from build123d import *

# Parameters (mm, degrees)
SKETCH4_R           = 36.068
BOSS_EXTRUDE1_DEPTH = 65.024
SKETCH5_R           = 21.463
BOSS_EXTRUDE2_DEPTH = 31.369


with BuildPart() as part:
    # Sketch1 → Revolve1 (revolve)
    with BuildSketch(Plane.XY, mode=Mode.PRIVATE) as revolve1_sk:
        Polygon((-70.612, -36.068), (-32.512, -36.068), (-32.512, -30.0863), (-70.612, -30.3149), align=None)
        Polygon((70.612, -30.3149), (32.512, -30.0863), (32.512, -36.068), (70.612, -36.068), align=None)
    revolve(revolve1_sk.sketch.rotate(Axis((-70.612, 0, 0), (1, 0, 0)), 270), axis=Axis((-70.612, 0, 0), (1, 0, 0)))



with BuildPart() as body_2:
    # Sketch2 → Revolve2 (revolve)
    with BuildSketch(Plane.XY):
        Polygon((16.8275, 59.944), (16.637, 31.369), (21.463, 31.369), (21.463, 59.944), align=None)
    revolve(axis=Axis((0, 0, 0), (0, 1, 0)))


with BuildPart() as part_1:
    add(part.part)

    add(body_2.part)  # Boss-Extrude1 merges body 2
    # Sketch4 → Boss-Extrude1 (add)
    with BuildSketch(Plane(origin=(-32.512, 0, 0), x_dir=(0, 0, -1), z_dir=(1, 0, 0))):
        with Locations(Location((0, 0, 0), (0, 0, 180))):
            Circle(SKETCH4_R)
    extrude(amount=BOSS_EXTRUDE1_DEPTH)

    # Sketch5 → Boss-Extrude2 (add)
    with BuildSketch(Plane.XZ.offset(-31.369)):
        Circle(SKETCH5_R)
    extrude(amount=BOSS_EXTRUDE2_DEPTH)

    # Sketch6 → Cut-Revolve1 (revolve, cut)
    with BuildSketch(Plane.XY, mode=Mode.PRIVATE) as cut_revolve1_sk:
        Polygon((-70.612, -30.3149), (-32.512, -30.0863), (-32.512, -24.6253), (32.512, -24.6253), (32.512, -30.0863), (70.612, -30.3149), (70.612, 0), (-70.612, 0), align=None)
    revolve(cut_revolve1_sk.sketch.rotate(Axis((70.612, 0, 0), (-1, 0, 0)), 270), axis=Axis((70.612, 0, 0), (-1, 0, 0)), mode=Mode.SUBTRACT)

    # Sketch7 → Cut-Revolve2 (revolve, cut)
    with BuildSketch(Plane.XY):
        Polygon((16.8275, 59.944), (16.637, 31.369), (12.1539, 31.369), (12.1539, 0), (0, 0), (0, 59.944), align=None)
    revolve(axis=Axis((0, 0, 0), (0, 1, 0)), mode=Mode.SUBTRACT)


solid = part_1.part
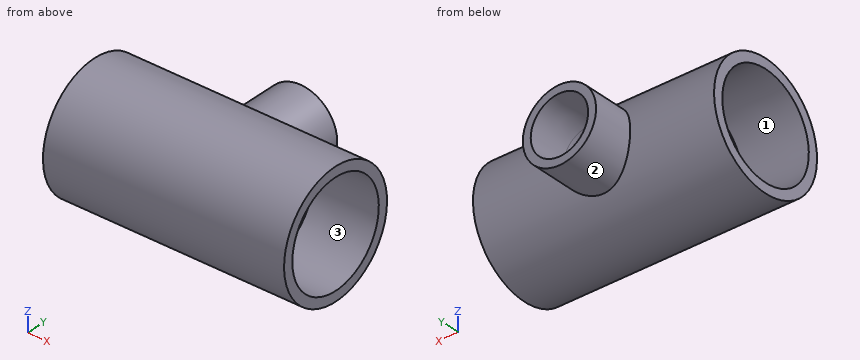
Can you work these out from the model? Positions are in its coordinate system, mm. Face numbers are marked on the shaded views. Coordinates: 2 decimals unless noted, no trailing zeros. Order: outer loops, then holes, each group sorted by start corner. A loop starts at its lowest first (then second) coordinate and runs counter-clockwise, first axis right, second up. Notation, with made-up numbers: (-24, 66) - (9, 66) arc R12 cw to (9, 72) - close; hole circle Ø10 at (-11, 80.5). An arc over 180 degrees is marked (long way). Answer as a JSON object with one key per item and string values. Group by question number.
Q1. I need wall thicknesses on line 1 (X direction, y = 26, z = 0); line 2 (Y direction, x = -11.5, z = 0); line 3 (Y direction, x = -36.5, z = 19). Which ranges of each line are inside material? Lowest first, please. Write a range as from..to.
Q2. Will these pins go through, and if not, where does the flat tip stop? P1, Ø5, axis at y = 9, z = -17.5, coming from the -X side (3 decimals); P2, Ø12, axis at x = 1.5, y = -17, coming from the +Z side; P3, Ø5, axis at x = 26.5, y = -13.5, coming from the -Z side; P4, Ø8, axis at x = -9, y = -6, coming from the -Z side.
Q3. We'd pull the mould along Z, two halves only. Please class the marked faces 1, 2 and 3: +Z half, -Z half, draft (parallel to the pull), parting line (faces both ways), or undercut.
Q4. Imagine slicing it at C-C (x = 35). Please give me the cut outline in (y, z).
Q5. Imagine slicing it at B-B (y = 46). Please give me the cut outline in (x, z), and give its area (3 significant figures).
Q6. Imagine slicing it at A-A (z = 0). Give the number of separate pieces and of enclosed holes in the cut face, and give its area (3 significant figures).
Determined:
{
 "1": {"line 1": "x = -32.51..-12.15, 12.15..32.51", "line 2": "y = -36.07..-24.63", "line 3": "y = -30.66..-23.36, 23.36..30.66"},
 "2": {"P1": "passes through", "P2": "stops at z = 34.35", "P3": "stops at z = -34.35", "P4": "stops at z = -36.01"},
 "3": {"face 1": "undercut", "face 2": "parting line", "face 3": "undercut"},
 "4": {"outline": "circle Ø72.14 at (0, 0); hole circle Ø60.2 at (0, 0)"},
 "5": {"outline": "circle Ø42.93 at (0, 0); hole circle Ø33.47 at (0, 0)", "area": "567 mm2"},
 "6": {"separate pieces": "3", "enclosed holes": "0", "area": "2,290 mm2"}
}
